from build123d import *

# Parameters (mm, degrees)
F1_DEPTH = 1.2


with BuildPart() as f1:
    # F0 (on Top) → F1 (new body)
    with BuildSketch(Plane.XY):
        with BuildLine():
            ThreePointArc((76.570266, -29.342705), (80.631141, -14.920425), (82, 0))
            ThreePointArc((82, 0), (46.647786, 67.438743), (-28.926442, 76.728489))
            ThreePointArc((-28.926442, 76.728489), (-48.410565, 66.18472), (-64.361077, 50.809958))
            ThreePointArc((-64.361077, 50.809958), (-58.139986, -57.825098), (50.459683, -64.636061))
            ThreePointArc((50.459683, -64.636061), (65.920841, -48.769281), (76.570266, -29.342705))
        make_face()
        with BuildLine():
            ThreePointArc((56.367426, 56.062138), (73.48966, 30.323585), (79.5, 0))
            ThreePointArc((79.5, 0), (-73.48966, -30.323585), (56.367426, 56.062138))
        make_face(mode=Mode.SUBTRACT)
        with BuildLine():
            ThreePointArc((-64.361077, 50.809958), (-48.410565, 66.18472), (-28.926442, 76.728489))
            ThreePointArc((-28.926442, 76.728489), (-54.306729, 74.245687), (-64.361077, 50.809958))
        make_face()
        with BuildLine():
            ThreePointArc((50.459683, -64.636061), (73.949669, -54.709135), (76.570266, -29.342705))
            ThreePointArc((76.570266, -29.342705), (65.920841, -48.769281), (50.459683, -64.636061))
        make_face()
    extrude(amount=F1_DEPTH)


solid = f1.part
Design review of the part built by this model. Coordinates are the model's own, in mm. Coordinates: 2 decimals unless noted, no trailing zeros. Write each loop counter-clockwise with the first axis right and the second up, starting at its lowest first coordinate (ties: lowest second). Pieces come first, ordered by that corner, then holes. Notation, with made-up numbers: (-1, 26) - (8, 26) arc R17 ccw to (8, 46) - close; hole circle Ø3 at (39, 45.5). An arc over 180 degrees is marked (long way). One line per item, written item: value.
1) To check wall thickness, follow probe 1 along Y at (x, z) = (0, 0.3); probe 2 along Y at (x, z) = (18, 0.1); probe 3 along X at (y, z) = (33.5, 0.75). State the ranges of each line that lie inside material, in increasing order.
Answer sheet:
probe 1: y = -82 to -79.5, 79.5 to 82
probe 2: y = -80 to -77.44, 77.44 to 80
probe 3: x = -74.84 to -72.1, 72.1 to 74.84
2) Add section B-B (y = -21). State the section outline as (x, z) points, plus the area to 3 significant figures.
Answer sheet:
outline: (-79.27, 0) - (-76.68, 0) - (-76.68, 1.2) - (-79.27, 1.2) - close; (76.68, 0) - (79.27, 0) - (79.27, 1.2) - (76.68, 1.2) - close
area: 6.21 mm2
3) Add section C-C (z = 0.6). State the section outline as (x, y) points.
Answer sheet:
outline: (-64.36, 50.81) arc R82 ccw to (50.46, -64.64) arc R25.05 ccw to (76.57, -29.34) arc R82 ccw to (82, 0) arc R82 ccw to (-28.93, 76.73) arc R25.05 ccw to start; hole (56.37, 56.06) arc R79.5 ccw (long way) to (79.5, 0) arc R79.5 ccw to start
4) Mouldability with a two-part tool opening along X and no side actions: class faces 1 (the face through (-54.003, 74.465, 0.592)), 2 (the face through (-13, 79, 0)) as +X half, -X half, draft (parallel to the pull), parting line (faces both ways), or undercut.
Answer sheet:
face 1: undercut
face 2: draft
5) Add section A-A (x = 0). State the section outline as (y, z) points.
Answer sheet:
outline: (-82, 0) - (-79.5, 0) - (-79.5, 1.2) - (-82, 1.2) - close; (79.5, 0) - (82, 0) - (82, 1.2) - (79.5, 1.2) - close
